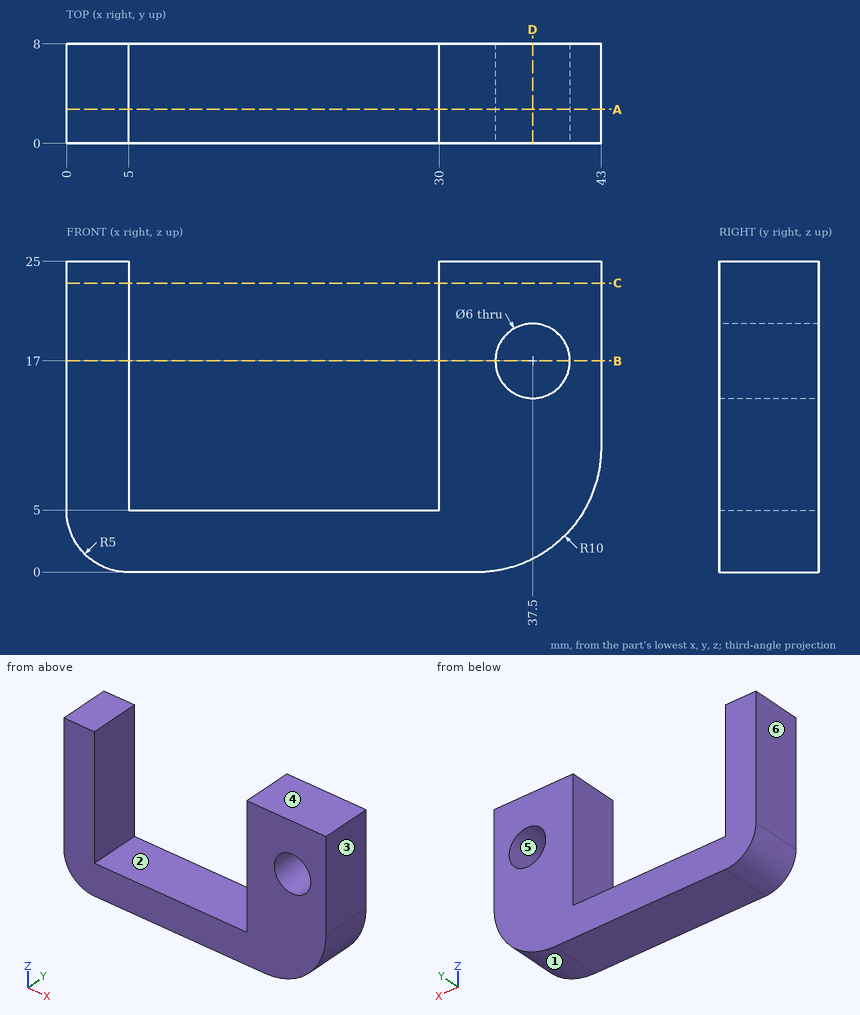
The drawing under review shows one solid part. Ordinate dimensions are in mm from its lowest x, y, z. A direction names the side the tool comes from. Give positions to 0.01 mm unless a question says otherwise; leave off trailing zeros. Write each loop counter-clockwise with the first axis right and the second up, starting at its lowest first coordinate (ties: lowest second). Pieces come first, ordered by that corner, then holes. Notation, with made-up numbers: (62, 40.5) - (80, 40.5) arc R24 cw to (80, 64.5) - close; hole circle Ø11 at (37.25, 17.5). An arc over 180 degrees is marked (long way). Answer in a Markdown table with one row per item. Add a question column.
1. We need section A-A on y = 2.75. Write out the cut boundary in (x, z).
2. We need section C-C on z = 23.25. Write out the cut boundary in (x, y).
3. Draft analysis for pull direction X (two halves, no side actions). For the marked faces 3, 4, 5 and 6, state which applies: +X half, -X half, draft (parallel to the pull), parting line (faces both ways), or undercut.
4. We need section B-B on z = 17. Write out the cut boundary in (x, y), then the cut area to 3 significant figures.
5. Tool access review of the marked faces 1 and 2: name each direction out of +Z, -Z, +X, -X, +Y, -Y from which nothing blocks a thin tool from reaching the whole face with its end or side.
6. Wall thickness on line 1 along X through (y, z) = (4, 17); line 2 along X through (y, z) = (1.25, 19.75); line 3 along X through (y, z) = (4, 24): over which ranges is each line inside the solid? List them lowest first. Write a range as [from, to].
7. We need section D-D on x = 37.5. Write out the cut boundary in (y, z), then the cut area to 3 significant figures.
8. Insertion check: P1, Ø5.5, axis at x = 37.5, z = 17, coming from the +Y side (3 decimals); P2, Ø1.5, axis at x = 13.5, y = 5, coming from the +Z side; P3, Ø12, axis at x = 29.5, z = 21, coming from the -Y side. Each pin has a flat end and moves straight along its axis. Give the tip position at first contact, or say it passes through.
Ans:
| question | item | result |
|---|---|---|
| 1 | outline | (0, 5) arc R5 ccw to (5, 0) - (33, 0) arc R10 ccw to (43, 10) - (43, 25) - (30, 25) - (30, 5) - (5, 5) - (5, 25) - (0, 25) - close; hole circle Ø6 at (37.5, 17) |
| 2 | outline | (0, 0) - (5, 0) - (5, 8) - (0, 8) - close; (30, 0) - (43, 0) - (43, 8) - (30, 8) - close |
| 3 | face 3 | +X half |
| 3 | face 4 | draft |
| 3 | face 5 | undercut |
| 3 | face 6 | -X half |
| 4 | outline | (0, 0) - (5, 0) - (5, 8) - (0, 8) - close; (30, 0) - (34.5, 0) - (34.5, 8) - (30, 8) - close; (40.5, 0) - (43, 0) - (43, 8) - (40.5, 8) - close |
| 4 | area | 96.0 mm^2 |
| 5 | face 1 | -Z, +X, +Y, -Y |
| 5 | face 2 | +Z, +Y, -Y |
| 6 | line 1 | x = [0, 5], [30, 34.5], [40.5, 43] |
| 6 | line 2 | x = [0, 5], [30, 36.3], [38.7, 43] |
| 6 | line 3 | x = [0, 5], [30, 43] |
| 7 | outline | (0, 1.07) - (8, 1.07) - (8, 14) - (0, 14) - close; (0, 20) - (8, 20) - (8, 25) - (0, 25) - close |
| 7 | area | 143 mm^2 |
| 8 | P1 | passes through |
| 8 | P2 | stops at z = 5 |
| 8 | P3 | stops at y = 0 |
